Read the model definition and answer for the solid it produces. Units are mm, in the model's axes. A direction names the side the tool comes from. Give positions to 0.01 mm unless a question says otherwise; leave off trailing zeros. Loops run counter-clockwise (first coordinate to the right, second up) from the corner with the lowest first, then second, coordinate; pieces in that order, holes last. Notation, with made-up numbers: (22, 88) - (75, 88) arc R31 ccw to (75, 123) - close; hole circle Ø10 at (40, -22). An arc over 180 degrees is marked (long way). Use a Markdown table: item, result. Add a question column.
Item 1: Which of the six approach directions +Z, -Z, +X, -X, +Y, -Y give full straight-line access (tool end or side, diameter ignored) to faces 5 (the face through (0, 1, -41)), 6 (the face through (-35, 2, -20))?
Item 2: A cutting plane is placed at C-C (y = 1.05). Determine the outline of the cut face in (x, z).
Item 3: For a pull along X with two mould halves and no side action, classify faces 1 (the face through (-40, 1, -39)), 2 (the face through (-5, 2, -20)), 3 (the face through (-20, 2, -45)), 4 (the face through (-20, 1, 0)) as +X half, -X half, draft (parallel to the pull), parting line (faces both ways), or undercut.
Item 4: A cutting plane is placed at A-A (x = -23.5). Determine the outline of the cut face in (y, z).
Item 5: A cutting plane is placed at B-B (z = -14.5). Determine the outline of the cut face in (x, y).
Item 6: Consider probe 1 along Z at (x, y) = (-18, 0.7); probe 2 along X at (y, z) = (0.95, -61). Determine where each line is inside the solid, lowest interval first. Write a range as [from, to].
Autodesk Inventor part; units mm, degrees
ref_plane "YZ Plane" through (0, 0, 0) normal (1, 0, 0) x (0, 1, 0)
ref_plane "XZ Plane" through (0, 0, 0) normal (0, 1, 0) x (-1, 0, 0)
ref_plane "XY Plane" through (0, 0, 0) normal (0, 0, 1) x (1, 0, 0)
sketch "Sketch1" plane through (0, 0, 0) normal (0, 1, 0) x (-1, 0, 0)
  line L0 (0, 0) -> (40, 0)
  line L1 (40, 0) -> (40, -80)
  line L2 (40, -80) -> (0, -80)
  line L3 (0, -80) -> (0, 0)
  dimension "d0" = 40
  dimension "d1" = 80
extrude "Extrusion1" add sketch "Sketch1" along normal blind 3
sketch "Sketch3" plane through (0, 3, 0) normal (0, 1, 0) x (1, 0, 0)
  line L0 (-40, 0) -> (0, 0)
  line L1 (-40, 0) -> (-40, 5)
  line L2 (-35, 5) -> (-5, 5)
  line L3 (0, 5) -> (0, 35)
  line L4 (0, 0) -> (0, 80)
  line L5 (-5, 35) -> (-35, 35)
  line L6 (-40, 80) -> (-40, 0)
  line L7 (-40, 35) -> (-40, 45)
  line L8 (0, 45) -> (-35, 45)
  line L9 (0, 45) -> (0, 75)
  line L10 (-5, 75) -> (-35, 75)
  line L11 (0, 80) -> (-40, 80)
  line L12 (-40, 80) -> (-35, 80)
  line L13 (0, 80) -> (-5, 80)
  line L14 (-5, 75) -> (-5, 45)
  line L15 (-5, 35) -> (-5, 5)
  line L16 (-35, 75) -> (-35, 45)
  line L17 (-35, 35) -> (-35, 5)
  dimension "d4" = 5
  dimension "d5" = 30
  dimension "d6" = 10
  dimension "d7" = 30
  dimension "d8" = 5
  dimension "d9" = 5
extrude "Extrusion2" cut sketch "Sketch3" against normal through all contours L8 L16 L10 L14 | L17 L5 L15 L2
properties part number "ClawExtender"
Geometry says:
| question | item | result |
|---|---|---|
| 1 | face 5 | +Z, -Z, +X, +Y, -Y |
| 1 | face 6 | +Y, -Y |
| 2 | outline | (-40, -80) - (0, -80) - (0, 0) - (-40, 0) - close; hole (-35, -75) - (-5, -75) - (-5, -45) - (-35, -45) - close; hole (-35, -35) - (-5, -35) - (-5, -5) - (-35, -5) - close |
| 3 | face 1 | -X half |
| 3 | face 2 | undercut |
| 3 | face 3 | undercut |
| 3 | face 4 | draft |
| 4 | outline | (0, -80) - (3, -80) - (3, -75) - (0, -75) - close; (0, -45) - (3, -45) - (3, -35) - (0, -35) - close; (0, -5) - (3, -5) - (3, 0) - (0, 0) - close |
| 5 | outline | (-40, 0) - (-35, 0) - (-35, 3) - (-40, 3) - close; (-5, 0) - (0, 0) - (0, 3) - (-5, 3) - close |
| 6 | probe 1 | [-80, -75], [-45, -35], [-5, 0] |
| 6 | probe 2 | [-40, -35], [-5, 0] |
